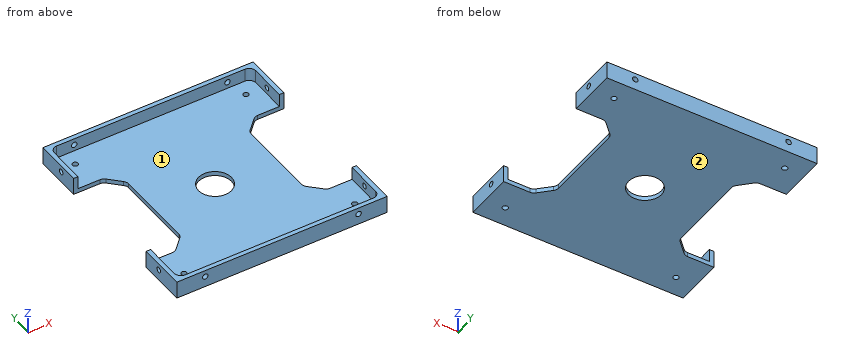
```python
from build123d import *

# Parameters (mm, degrees)
SKETCH1_W                      = 96
SKETCH1_H                      = 96
BOSS_EXTRUDE1_DEPTH            = 8
SKETCH2_W                      = 92
SKETCH2_H                      = 92
COMPONENT_PLATFORM_DEPTH       = 6
CABLE_SLOTS_DEPTH              = 6
SKETCH4_R                      = 7.5
CENTER_MASS_CUT_DEPTH          = 6
INNER_CORNER_FILLETS_R         = 3
M3X0_5_TAPPED_HOLE1_AT_2_COUNT = 2
M3X0_5_TAPPED_HOLE1_AT_2_PITCH = 70
M3X0_5_TAPPED_HOLE2_AT_2_COUNT = 2
M3X0_5_TAPPED_HOLE2_AT_2_PITCH = 70
M3X0_5_TAPPED_HOLE3_D          = 2.5
M3X0_5_TAPPED_HOLE3_DEPTH      = 10
M3X0_5_TAPPED_HOLE3_TIP        = 0.751075774


with BuildPart() as part:
    # Sketch1 → Boss-Extrude1 (new body)
    with BuildSketch(Plane.XY):
        Rectangle(SKETCH1_W, SKETCH1_H)
    extrude(amount=BOSS_EXTRUDE1_DEPTH)

    # Sketch2 → Component Platform (cut)
    with BuildSketch(Plane.XY.offset(8)):
        Rectangle(SKETCH2_W, SKETCH2_H)
    extrude(amount=-COMPONENT_PLATFORM_DEPTH, mode=Mode.SUBTRACT)

    # Sketch3 → Cable Slots (cut, symmetric)
    with BuildSketch(Plane.XY.offset(2)):
        with BuildLine():
            Line((-33.878679656, -25.121320344), (-28.878679656, -20.121320344))
            ThreePointArc((-28.878679656, -20.121320344), (-28.228361402, -19.148050297), (-28, -18))
            Line((-28, -18), (-28, 18))
            ThreePointArc((-28, 18), (-28.228361402, 19.148050297), (-28.878679656, 20.121320344))
            Line((-28.878679656, 20.121320344), (-33.878679656, 25.121320344))
            ThreePointArc((-33.878679656, 25.121320344), (-34.851949703, 25.771638598), (-36, 26))
            Line((-36, 26), (-48, 26))
            Line((-48, 26), (-48, -26))
            Line((-48, -26), (-36, -26))
            ThreePointArc((-36, -26), (-34.851949703, -25.771638598), (-33.878679656, -25.121320344))
        make_face()
        with BuildLine():
            Line((48, -26), (48, 26))
            Line((48, 26), (36, 26))
            ThreePointArc((36, 26), (34.851949703, 25.771638598), (33.878679656, 25.121320344))
            Line((33.878679656, 25.121320344), (28.878679656, 20.121320344))
            ThreePointArc((28.878679656, 20.121320344), (28.228361402, 19.148050297), (28, 18))
            Line((28, 18), (28, -18))
            ThreePointArc((28, -18), (28.228361402, -19.148050297), (28.878679656, -20.121320344))
            Line((28.878679656, -20.121320344), (33.878679656, -25.121320344))
            ThreePointArc((33.878679656, -25.121320344), (34.851949703, -25.771638598), (36, -26))
            Line((36, -26), (48, -26))
        make_face()
    extrude(amount=CABLE_SLOTS_DEPTH, both=True, mode=Mode.SUBTRACT)

    # Sketch4 → Center Mass Cut (cut)
    with BuildSketch(Plane.XY.offset(2)):
        Circle(SKETCH4_R)
    extrude(amount=-CENTER_MASS_CUT_DEPTH, mode=Mode.SUBTRACT)

    # Inner Corner Fillets
    inner_corner_fillets_edges = [part.edges().sort_by_distance(p)[0] for p in [
        (-46, -46, 5),
        (-46, 46, 5),
        (46, 46, 5),
        (46, -46, 5),
    ]]
    fillet(inner_corner_fillets_edges, radius=INNER_CORNER_FILLETS_R)

    # Sketch11 → M3x0.5 Tapped Hole1 (revolve, cut)
    with BuildSketch(Plane(origin=(-35, -48, 5), x_dir=(0, 0, -1), z_dir=(1, 0, 0))):
        Polygon((0, 0), (0, 10.751075774), (1.25, 10), (1.25, 0), align=None)
    m3x0_5_tapped_hole1 = revolve(axis=Axis((-35, -54.35, 5), (0, 1, 0)), mode=Mode.SUBTRACT)

    # M3x0.5 Tapped Hole1 at 2: M3x0.5 Tapped Hole1 ×2
    with Locations(*[(i * M3X0_5_TAPPED_HOLE1_AT_2_PITCH, 0, 0) for i in range(1, M3X0_5_TAPPED_HOLE1_AT_2_COUNT)]):
        add(m3x0_5_tapped_hole1, mode=Mode.SUBTRACT)

    # Sketch13 → M3x0.5 Tapped Hole2 (revolve, cut)
    with BuildSketch(Plane(origin=(48, -35, 5), x_dir=(0, 0, -1), z_dir=(0, 1, 0))):
        Polygon((0, 0), (0, 10.751075774), (1.25, 10), (1.25, 0), align=None)
    m3x0_5_tapped_hole2 = revolve(axis=Axis((54.35, -35, 5), (-1, 0, 0)), mode=Mode.SUBTRACT)

    # M3x0.5 Tapped Hole2 at 2: M3x0.5 Tapped Hole2 ×2
    with Locations(*[(0, i * M3X0_5_TAPPED_HOLE2_AT_2_PITCH, 0) for i in range(1, M3X0_5_TAPPED_HOLE2_AT_2_COUNT)]):
        add(m3x0_5_tapped_hole2, mode=Mode.SUBTRACT)

    # Mirror1: M3x0.5 Tapped Hole1 across plane
    add(m3x0_5_tapped_hole1.mirror(Plane(origin=(0, 0, 0), x_dir=(0, 0, 1), z_dir=(0, -1, 0))), mode=Mode.SUBTRACT)

    # Mirror1 copy 1 sketch → Mirror1 copy 1 (revolve, cut)
    with BuildSketch(Plane(origin=(35, 48, 5), x_dir=(0, 0, -1), z_dir=(1, 0, 0))):
        Polygon((0, 0), (0, -10.751075774), (1.25, -10), (1.25, 0), align=None)
    revolve(axis=Axis((35, 54.35, 5), (0, 1, 0)), mode=Mode.SUBTRACT)

    # Mirror2: M3x0.5 Tapped Hole2 across plane
    add(m3x0_5_tapped_hole2.mirror(Plane(origin=(0, 0, 0), x_dir=(0, 0, 1), z_dir=(1, 0, 0))), mode=Mode.SUBTRACT)

    # Mirror2 copy 1 sketch → Mirror2 copy 1 (revolve, cut)
    with BuildSketch(Plane(origin=(-48, 35, 5), x_dir=(0, 0, -1), z_dir=(0, 1, 0))):
        Polygon((0, 0), (0, -10.751075774), (1.25, -10), (1.25, 0), align=None)
    revolve(axis=Axis((-54.35, 35, 5), (-1, 0, 0)), mode=Mode.SUBTRACT)

    # M3x0.5 Tapped Hole3
    with Locations(Plane.XY.offset(2)):
        with Locations((-39, -39), (39, -39), (39, 39), (-39, 39)):
            Hole(M3X0_5_TAPPED_HOLE3_D / 2, depth=M3X0_5_TAPPED_HOLE3_DEPTH)
            with Locations((0, 0, -(M3X0_5_TAPPED_HOLE3_DEPTH + M3X0_5_TAPPED_HOLE3_TIP / 2))):  # 118° drill point
                Cone(0, M3X0_5_TAPPED_HOLE3_D / 2, M3X0_5_TAPPED_HOLE3_TIP, mode=Mode.SUBTRACT)


solid = part.part
```
Could you check a few things on this model? Use its own coordinates, in mm. Face numbers are marked on the shaded views. Give positions to 0.01 mm unless a question says otherwise; leave off trailing zeros. Loops run counter-clockwise (first coordinate to the right, second up) from the corner with the lowest first, then second, coordinate; pieces in that order, holes last. Notation, with made-up numbers: (77, 64) -> (135, 64) arc R22 cw to (135, 78) -> close; hole circle Ø10 at (-25, -25.5). An arc over 180 degrees is marked (long way). Put each result on its own line as item: value.
(1) Please list where these lines run through material, in increasing order: probe 1 along X at (y, z) = (47.3, 5); probe 2 along Y at (x, z) = (-47.6, 5); probe 3 along Y at (x, z) = (39, 1.1). Write a range as [from, to].
Computed:
probe 1: [-48, -36.25], [-33.75, 33.75], [36.25, 48]
probe 2: [-48, -36.25], [-33.75, -26], [26, 33.75], [36.25, 48]
probe 3: [-48, -40.25], [-37.75, -26], [26, 37.75], [40.25, 48]
(2) Imagine slicing it at B-B on x = 39. Write out the boundary of the cut face in (y, z).
Computed:
outline: (-48, 0) -> (-40.25, 0) -> (-40.25, 2) -> (-46, 2) -> (-46, 8) -> (-48, 8) -> close; (-37.75, 0) -> (-26, 0) -> (-26, 2) -> (-37.75, 2) -> close; (26, 0) -> (37.75, 0) -> (37.75, 2) -> (26, 2) -> close; (40.25, 0) -> (48, 0) -> (48, 8) -> (46, 8) -> (46, 2) -> (40.25, 2) -> close
(3) Imagine slicing it at C-C on y = -35. Write out the boundary of the cut face in (x, z).
Computed:
outline: (-48, 0) -> (48, 0) -> (48, 3.75) -> (46, 3.75) -> (46, 2) -> (-46, 2) -> (-46, 3.75) -> (-48, 3.75) -> close; (-48, 6.25) -> (-46, 6.25) -> (-46, 8) -> (-48, 8) -> close; (46, 6.25) -> (48, 6.25) -> (48, 8) -> (46, 8) -> close
(4) Imagine slicing it at D-D on x = 0. Write out the boundary of the cut face in (y, z), plus the area to 3 significant figures.
Computed:
outline: (-48, 0) -> (-7.5, 0) -> (-7.5, 2) -> (-46, 2) -> (-46, 8) -> (-48, 8) -> close; (7.5, 0) -> (48, 0) -> (48, 8) -> (46, 8) -> (46, 2) -> (7.5, 2) -> close
area: 186 mm^2
(5) Thinking about a two-plate mould opening in Y: for the marked faces 1 and 2, which applies, pulls with the +Y half, pulls with the -Y half, needs draft (parallel to the pull), parting line crosses it, or undercut?
Computed:
face 1: undercut
face 2: needs draft
(6) Imagine slicing it at A-A on y = 0. Write out the boundary of the cut face in (x, z), plus the area to 3 significant figures.
Computed:
outline: (-28, 0) -> (-7.5, 0) -> (-7.5, 2) -> (-28, 2) -> close; (7.5, 0) -> (28, 0) -> (28, 2) -> (7.5, 2) -> close
area: 82.0 mm^2
(7) I'm going to push flat-ended pins straight in: pin 1 Ø3 at (x, z) = (35, 5) entering from -Y; pin 2 Ø1 at (x, y) = (-26, 10.5) entering from +Z; pin 3 Ø2 at (y, z) = (-4.5, 1.5) entering from -X; pin 4 Ø1.6 at (y, z) = (-8, 0.5) entering from +X. Where does each tip first touch, or does it pass through?
Computed:
pin 1: y = -48
pin 2: z = 2
pin 3: x = -28
pin 4: x = 28
